Verification items for the finished model (mm, model axes). Give positions to 0.01 mm unless a question says otherwise; leave off trailing zeros. Order: outer loops, then holes, each group sorted by start corner. A loop starts at its lowest first (then second) coordinate and runs counter-clockwise, first axis right, second up. Notation, with made-up numbers: (-23.75, 83) - (-16.75, 83) arc R8 ccw to (-16.75, 92) - close; hole circle Ø2 at (10.5, 40). An arc over 180 degrees is marked (long way). Answer as a JSON object with one key per item and string values.
```python
from build123d import *

# Parameters (mm, degrees)
SKETCH1_W           = 10
SKETCH1_H           = 10
SKETCH1_W_2         = 8
SKETCH1_H_2         = 8
BOSS_EXTRUDE1_DEPTH = 600
FILLET1_R           = 1
FILLET2_R           = 1


with BuildPart() as part:
    # Sketch1 → Boss-Extrude1 (new body)
    with BuildSketch(Plane.XY):
        with Locations((-2.879581152, 1.714659686)):
            Rectangle(SKETCH1_W, SKETCH1_H)
        with Locations((-2.879581152, 1.714659686)):
            Rectangle(SKETCH1_W_2, SKETCH1_H_2, mode=Mode.SUBTRACT)
    extrude(amount=BOSS_EXTRUDE1_DEPTH)

    # Fillet1
    fillet1_edges = [part.edges().sort_by_distance(p)[0] for p in [
        (-6.879581152, -2.285340314, 300),
        (2.120418848, -3.285340314, 300),
        (-7.879581152, 6.714659686, 300),
        (2.120418848, 6.714659686, 300),
    ]]
    fillet(fillet1_edges, radius=FILLET1_R)

    # Fillet2
    fillet2_edges = [part.edges().sort_by_distance(p)[0] for p in [
        (1.120418848, -2.285340314, 300),
        (1.120418848, 5.714659686, 300),
        (-6.879581152, 5.714659686, 300),
        (-7.879581152, -3.285340314, 300),
    ]]
    fillet(fillet2_edges, radius=FILLET2_R)


solid = part.part
```
(1) Section check C-C (x = -1.75). Record the cut outline in (y, z).
Computed values:
{"outline": "(-3.29, 0) - (-2.29, 0) - (-2.29, 600) - (-3.29, 600) - close; (5.71, 0) - (6.71, 0) - (6.71, 600) - (5.71, 600) - close"}
(2) Material ranges on line 1 along X through (y, z) = (3.5, 377.5); line 2 along Y through (x, z) = (-3, 172.5); line 3 along Y through (x, z) = (0.5, 467), recorded low to high. Write a range as [from, to].
Computed values:
{"line 1": "x = [-7.88, -6.88], [1.12, 2.12]", "line 2": "y = [-3.29, -2.29], [5.71, 6.71]", "line 3": "y = [-3.29, -2.21], [5.64, 6.71]"}
(3) Section check B-B (z = 371.5). Record the cut outline in (x, y).
Computed values:
{"outline": "(-7.88, -2.29) arc R1 ccw to (-6.88, -3.29) - (1.12, -3.29) arc R1 ccw to (2.12, -2.29) - (2.12, 5.71) arc R1 ccw to (1.12, 6.71) - (-6.88, 6.71) arc R1 ccw to (-7.88, 5.71) - close; hole (-6.88, -1.29) arc R1 ccw to (-5.88, -2.29) - (0.12, -2.29) arc R1 ccw to (1.12, -1.29) - (1.12, 4.71) arc R1 ccw to (0.12, 5.71) - (-5.88, 5.71) arc R1 ccw to (-6.88, 4.71) - close"}
(4) Section check A-A (y = 2.5). Record the cut outline in (x, z).
Computed values:
{"outline": "(-7.88, 0) - (-6.88, 0) - (-6.88, 600) - (-7.88, 600) - close; (1.12, 0) - (2.12, 0) - (2.12, 600) - (1.12, 600) - close"}
